Geometry: final body of the model. Coordinates: model frame, mm. A direction names the side the tool comes from. Coordinates: 2 decimals unless noted, no trailing zeros. Loops run counter-clockwise (first coordinate to the right, second up) from the corner with the lowest first, then second, coordinate; pieces in that order, holes last. Notation, with made-up numbers: M 29.25,89.5 L 67.25,89.5 A5 ccw 67.25,97.5 Z; hole C 29,-14.5 d2. An arc over 180 degrees is marked long. Write each question's results on one line, items separated by ' | '. Start each with the question number.
from build123d import *

# Parameters (mm, degrees)
BOX004_W          = 20
BOX004_H          = 2
BOX004_DEPTH      = 14.5
BOX004_ROLL_ANGLE = 45
BOX001_W          = 20
BOX001_H          = 30
BOX001_DEPTH      = 34
BOX_W             = 20
BOX_H             = 24
BOX_DEPTH         = 38
BOX002_W          = 20
BOX002_H          = 18
BOX002_DEPTH      = 8
BOX003_W          = 20
BOX003_H          = 20
BOX003_DEPTH      = 10
FILLET_R          = 0.5


with BuildPart() as cube004:
    # Box004 → Box004 (new body)
    with BuildSketch(Plane.XY):
        with Locations((10, 1)):
            Rectangle(BOX004_W, BOX004_H)
    extrude(amount=BOX004_DEPTH)


with BuildPart() as cube004_1:
    # Box004 roll: moved
    add(cube004.part.rotate(Axis((0, 0, 0), (1, 0, 0)), BOX004_ROLL_ANGLE))


with BuildPart() as cube004_2:
    # Box004 placement: moved
    add(cube004_1.part.moved(Location((0, 0, 10))))


with BuildPart() as cube001:
    # Box001 → Box001 (new body)
    with BuildSketch(Plane(origin=(0, 2, 2), x_dir=(1, 0, 0), z_dir=(0, 0, 1))):
        with Locations((10, 15)):
            Rectangle(BOX001_W, BOX001_H)
    extrude(amount=BOX001_DEPTH)


with BuildPart() as cut:
    # Box → Box (new body)
    with BuildSketch(Plane.XY):
        with Locations((10, 12)):
            Rectangle(BOX_W, BOX_H)
    extrude(amount=BOX_DEPTH)

    # Cut: cut Cube001
    add(cube001.part, mode=Mode.SUBTRACT)


with BuildPart() as cube002:
    # Box002 → Box002 (new body)
    with BuildSketch(Plane(origin=(0, -18, 22), x_dir=(1, 0, 0), z_dir=(0, 0, 1))):
        with Locations((10, 9)):
            Rectangle(BOX002_W, BOX002_H)
    extrude(amount=BOX002_DEPTH)


with BuildPart() as fillet_body:
    # Box003 → Box003 (new body)
    with BuildSketch(Plane(origin=(0, -20, 20), x_dir=(1, 0, 0), z_dir=(0, 0, 1))):
        with Locations((10, 10)):
            Rectangle(BOX003_W, BOX003_H)
    extrude(amount=BOX003_DEPTH)

    # Cut001: cut Cube002
    add(cube002.part, mode=Mode.SUBTRACT)

    # Fusion: union Cut
    add(cut.part)

    # Fusion001: union Cube004
    add(cube004_2.part)

    # Fillet
    fillet_edges = [fillet_body.edges().sort_by_distance(p)[0] for p in [
        (10, -20, 30),
        (10, -20, 20),
        (10, 0, 38),
        (10, 24, 38),
        (10, 24, 36),
        (10, 24, 2),
        (10, 24, 0),
        (10, 0, 0),
    ]]
    fillet(fillet_edges, radius=FILLET_R)


solid = fillet_body.part
Item 1: Section D-D, the plane y = -8. Return loops of the section in (x, z), plus the area to 3 significant figures.
Item 2: Pull-direction query (Z, two-part tool) for faces 5 (the flat face through (9.86, -3.536, 16.364)), 6 (the flat face through (10, 12, 0)), 7 (the flat face through (10, 0, 16)), 8 (the flat face through (10, -18, 26)); classes: released by +Z, released by -Z, zero draft, split by the parting line, or undercut.
Item 3: Ray query, L1, parallel to Z at x = 14, y = 8; L2, parallel to Y at x = 15.5, z = 21; L3, parallel to Z at x = 5.25, y = -11. Return the intervals inside material, ascending. Write a range as [from, to].
Item 4: Set-up query: faces 1 (the flat face through (10, -19, 30)), 2 (the flat face through (10, -4, 20)), 3 (the flat face through (10, -9, 22)), 4 (the flat face through (10, 13, 2)). Return all of +Z, -Z, +X, -X, +Y, -Y with unobstructed straight access to the full face (end or side cutting, diameter ignored); none if empty.
Item 5: Section A-A, the plane y = 10.5. Return loops of the section in (x, z).
Item 6: Section C-C, the plane z = 17. Return loops of the section in (x, y).
Item 7: Contact query for flat-ended pins moving along their axis: P1, Ø3.5, axis at x = 8, z = 18, coming from the -Y side; P2, Ø3, axis at x = 10.5, z = 6.5, coming from the -Y side; P3, Ø10.5, axis at x = 10, y = -13.5, coming from the -Z side. Output: stop coordinate, or through.
Item 8: Section B-B, the plane x = 14. Return loops of the section in (y, z), plus the area to 3 significant figures.
Solutions:
1) outline: M 0,18 L 20,18 L 20,22 L 0,22 Z | area: 80.0 mm²
2) face 5: undercut | face 6: released by -Z | face 7: undercut | face 8: zero draft
3) L1: z = [0, 2], [36, 38] | L2: y = [-20, 2] | L3: z = [20, 22]
4) face 1: +Z, +X, -X, -Y | face 2: +X, -X | face 3: +Z, +X, -X | face 4: +X, -X, +Y
5) outline: M 0,0 L 20,0 L 20,2 L 0,2 Z; M 0,36 L 20,36 L 20,38 L 0,38 Z
6) outline: M 0,-7 L 20,-7 L 20,-4.17 L 0,-4.17 Z; M 0,0 L 20,0 L 20,2 L 0,2 Z
7) P1: stops at y = -9.75 | P2: stops at y = 0 | P3: stops at z = 18.25
8) outline: M -20,20.5 A0.5 ccw -19.5,20 L -10,20 L 0,10 L 0,0.5 A0.5 ccw 0.5,0 L 23.5,0 A0.5 ccw 24,0.5 L 24,1.5 A0.5 ccw 23.5,2 L 2,2 L 2,36 L 23.5,36 A0.5 ccw 24,36.5 L 24,37.5 A0.5 ccw 23.5,38 L 0.5,38 A0.5 ccw 0,37.5 L 0,22 L -18,22 L -18,30 L -19.5,30 A0.5 ccw -20,29.5 Z; hole M -7.17,20 L 0,12.83 L 0,20 Z | area: 244 mm²
